Source: CAD feature listing. Evaluate the final solid. Frame: model axes, mm. A direction names the side the tool comes from. Round coordinates to 2 decimals unless told otherwise and drop trailing zeros. Write each loop counter-clockwise with the first axis right and the second up, starting at its lowest first coordinate (ties: lowest second). Pieces come first, ordered by that corner, then holes. Notation, with made-up numbers: M 10.5,62.5 L 30.5,62.5 A9 cw 30.5,72.5 Z; hole C 57.5,39.5 d2. An arc over 180 degrees is marked long. Put each result on its own line as item: value. Start each with the question number.
```python
from build123d import *

# Parameters (mm, degrees)
EXTRUDE_1_DEPTH     = 1.6
SKETCH_2_R          = 1.5
CUT_EXTRUDE_1_DEPTH = 47.602172696
SKETCH_3_R          = 2.2
SKETCH_3_R_2        = 1.5
EXTRUDE_2_DEPTH     = 5
EXTRUDE_3_DEPTH     = 7
SKETCH_5_W          = 14
SKETCH_5_H          = 6
EXTRUDE_4_DEPTH     = 10
SKETCH_6_W          = 3
SKETCH_6_H          = 18
SKETCH_6_H_2        = 30
EXTRUDE_5_DEPTH     = 3
SKETCH_7_W          = 7
SKETCH_7_H          = 38.2
CUT_EXTRUDE_2_DEPTH = 4


with BuildPart() as part:
    # 草图1 → 凸台-拉伸1 (new body)
    with BuildSketch(Plane.XY):
        with BuildLine():
            Line((-34, -29.55), (34, -29.55))
            ThreePointArc((34, -29.55), (35.414213562, -28.964213562), (36, -27.55))
            Line((36, -27.55), (36, 27.55))
            ThreePointArc((36, 27.55), (35.414213562, 28.964213562), (34, 29.55))
            Line((34, 29.55), (-34, 29.55))
            ThreePointArc((-34, 29.55), (-35.414213562, 28.964213562), (-36, 27.55))
            Line((-36, 27.55), (-36, -27.55))
            ThreePointArc((-36, -27.55), (-35.414213562, -28.964213562), (-34, -29.55))
        make_face()
    extrude(amount=EXTRUDE_1_DEPTH)

    # 草图2 → 切除-拉伸1 (cut, through all)
    with BuildSketch(Plane.XY.offset(1.6)):
        with Locations((-33, 26.55)):
            Circle(SKETCH_2_R)
        with Locations((33, 26.55)):
            Circle(SKETCH_2_R)
        with Locations((-33, -19.65)):
            Circle(SKETCH_2_R)
        with Locations((33, -19.65)):
            Circle(SKETCH_2_R)
    extrude(amount=-CUT_EXTRUDE_1_DEPTH, mode=Mode.SUBTRACT)

    # 草图3 → 凸台-拉伸2 (add)
    # profile 1 of 4: a face of its own
    with BuildSketch(Plane(origin=(0, 0, 0), x_dir=(-1, 0, 0), z_dir=(0, 0, -1))):
        with Locations((33, 26.55)):
            Circle(SKETCH_3_R)
        with Locations(Location((33, 26.55, 0), (0, 0, 180))):
            Circle(SKETCH_3_R_2, mode=Mode.SUBTRACT)
    # profile 2 of 4: a face of its own
    with BuildSketch(Plane(origin=(0, 0, 0), x_dir=(-1, 0, 0), z_dir=(0, 0, -1))):
        with Locations((33, -19.65)):
            Circle(SKETCH_3_R)
        with Locations(Location((33, -19.65, 0), (0, 0, 180))):
            Circle(SKETCH_3_R_2, mode=Mode.SUBTRACT)
    # profile 3 of 4: a face of its own
    with BuildSketch(Plane(origin=(0, 0, 0), x_dir=(-1, 0, 0), z_dir=(0, 0, -1))):
        with Locations((-33, -19.65)):
            Circle(SKETCH_3_R)
        with Locations(Location((-33, -19.65, 0), (0, 0, 180))):
            Circle(SKETCH_3_R_2, mode=Mode.SUBTRACT)
    # profile 4 of 4: a face of its own
    with BuildSketch(Plane(origin=(0, 0, 0), x_dir=(-1, 0, 0), z_dir=(0, 0, -1))):
        with Locations((-33, 26.55)):
            Circle(SKETCH_3_R)
        with Locations(Location((-33, 26.55, 0), (0, 0, 180))):
            Circle(SKETCH_3_R_2, mode=Mode.SUBTRACT)
    extrude(amount=EXTRUDE_2_DEPTH)

    # 草图4 → 凸台-拉伸3 (add)
    with BuildSketch(Plane.XY.offset(1.6)):
        Polygon((-29, 29.55), (-29, 22.55), (-36, 22.55), (-36, -15.65), (-29, -15.65), (-29, -29.55), (29, -29.55), (29, -15.65), (36, -15.65), (36, 22.55), (29, 22.55), (29, 29.55), align=None)
    extrude(amount=EXTRUDE_3_DEPTH)

    # 草图5 → 凸台-拉伸4 (add)
    with BuildSketch(Plane(origin=(0, 0, 0), x_dir=(-1, 0, 0), z_dir=(0, 0, -1))):
        with Locations((27, -26.55)):
            Rectangle(SKETCH_5_W, SKETCH_5_H)
    extrude(amount=EXTRUDE_4_DEPTH)

    # 草图6 → 凸台-拉伸5 (add)
    with BuildSketch(Plane.XY.offset(1.6)):
        with Locations((-37.5, 13.55)):
            Rectangle(SKETCH_6_W, SKETCH_6_H)
        with Locations((37.5, 5.55)):
            Rectangle(SKETCH_6_W, SKETCH_6_H_2)
    extrude(amount=EXTRUDE_5_DEPTH)

    # 草图7 → 切除-拉伸2 (cut)
    with BuildSketch(Plane.XY.offset(8.6)):
        with Locations((32.5, 3.45)):
            Rectangle(SKETCH_7_W, SKETCH_7_H)
    extrude(amount=-CUT_EXTRUDE_2_DEPTH, mode=Mode.SUBTRACT)


solid = part.part
```
(1) Access query for faces 1 (the flat face through (-33, -23, 1.6)), 2 (the flat face through (32, -15.65, 3)), 3 (the flat face through (34, 4, 4.6)), 4 (the flat face through (-32, 25, -5)). Directions: +Z, -Z, +X, -X, +Y, -Y. A direction counts if a zero-diameter tool reaches every point of the face in a straight line with its end or side. Return the directions, or none.
(2) Section query C-C (y = 18.5). Return loops of the section in (x, z), and give its area (3 significant figures).
(3) Section query B-B (x = 33). Return loops of the section in (y, z).
(4) Section query A-A (y = 26.55). Return loops of the section in (x, z).
(5) Section query D-D (z = -6.5). Return loops of the section in (x, y), and give its area (3 significant figures).
(6) Ray query, line 1 along X through (y, z) = (26.5, 0.5); line 2 along Y through (x, z) = (-33, 0.5); line 3 along Z through (x, y) = (35, 10.5). Return the intervals inside material, ascending.
(7) Contact query for flat-ended pins moving along their axis: P1, Ø5, axis at y = -19, z = -3.5, coming from the +X side; P2, Ø5, axis at x = -26, z = -3.5, coming from the +Y side; P3, Ø3.5, axis at x = 32, y = 26.5, coming from the -Z side. Output: stop coordinate, or through.
(8) Pull-direction query (Y, two-part tool) for faces 5 (the flat face through (-38, 4.55, 3)), 6 (the flat face through (36, 0, 1)), 7 (the cylindrical face through (35.2, 26.6, -2.5)); classes: +Y half, -Y half, draft (parallel to the pull), parting line (faces both ways), or undercut.
Entries:
1. face 1: +Z, -X, -Y
1. face 2: +Z, +X, -Y
1. face 3: +Z, +X, +Y, -Y
1. face 4: -Z, +X, -X, +Y
2. outline: M -39,1.6 L -36,1.6 L -36,0 L 36,0 L 36,1.6 L 39,1.6 L 39,4.6 L 29,4.6 L 29,8.6 L -36,8.6 L -36,4.6 L -39,4.6 Z
2. area: 609 mm2
3. outline: M -29.55,0 L -21.85,0 L -21.85,-5 L -21.15,-5 L -21.15,1.6 L -29.55,1.6 Z; M -18.15,-5 L -17.45,-5 L -17.45,0 L 24.35,0 L 24.35,-5 L 25.05,-5 L 25.05,1.6 L 22.55,1.6 L 22.55,4.6 L -15.65,4.6 L -15.65,1.6 L -18.15,1.6 Z; M 28.05,-5 L 28.75,-5 L 28.75,0 L 29.55,0 L 29.55,1.6 L 28.05,1.6 Z
4. outline: M -36,0 L -35.2,0 L -35.2,-5 L -34.5,-5 L -34.5,1.6 L -36,1.6 Z; M -31.5,-5 L -30.8,-5 L -30.8,0 L 30.8,0 L 30.8,-5 L 31.5,-5 L 31.5,1.6 L 29,1.6 L 29,8.6 L -29,8.6 L -29,1.6 L -31.5,1.6 Z; M 34.5,-5 L 35.2,-5 L 35.2,0 L 36,0 L 36,1.6 L 34.5,1.6 Z
5. outline: M -34,-29.55 L -20,-29.55 L -20,-23.55 L -34,-23.55 Z
5. area: 84.0 mm2
6. line 1: -36 to -34.5, -31.5 to 31.5, 34.5 to 36
6. line 2: -29.55 to -21.15, -18.15 to 25.05, 28.05 to 29.55
6. line 3: 0 to 4.6
7. P1: x = 35.2
7. P2: y = -23.55
7. P3: z = -5
8. face 5: -Y half
8. face 6: draft
8. face 7: undercut
